Could you check a few things on this model? Use its own coordinates, in mm. A direction names the side the tool comes from. Give positions to 0.01 mm unless a question says otherwise; leave off trailing zeros. Write each loop counter-clockwise with the first axis right and the second up, starting at its lowest first coordinate (ties: lowest second). Pieces come first, ordered by that corner, then holes. Notation, with made-up numbers: (73, 0.25) - (104, 0.25) arc R19 cw to (104, 30.25) - close; hole circle Ø4 at (41.5, -33.75). An arc over 180 degrees is marked (long way). Answer in a Markdown table with one row per item.
Autodesk Inventor part; units mm, degrees
ref_plane "YZ Plane" through (0, 0, 0) normal (1, 0, 0) x (0, 1, 0)
ref_plane "XZ Plane" through (0, 0, 0) normal (0, 1, 0) x (-1, 0, 0)
ref_plane "XY Plane" through (0, 0, 0) normal (0, 0, 1) x (1, 0, 0)
sketch "Sketch1" plane through (0, 0, 0) normal (0, 0, 1) x (1, 0, 0)
  line L0 (33.401, 0) -> (-33.401, 0) construction
  arc A0 (38.9253, 5.6997) -> (35.7349, -7.5866) centre (33.401, 0) ccw construction
  arc A1 (-35.7349, -7.5866) -> (-38.9253, 5.6997) centre (-33.401, 0) ccw construction
  line L1 (19.1135, -12.7) -> (19.1135, -38.1)
  line L2 (-19.1135, -38.1) -> (-19.1135, -12.7)
  line L3 (-19.1135, -12.7) -> (-35.7349, -7.5866)
  arc A2 (35.7349, -7.5866) -> (38.9253, 5.6997) centre (33.401, 0) ccw
  arc A3 (-38.9253, 5.6997) -> (-35.7349, -7.5866) centre (-33.401, 0) ccw
  line L4 (0, 55.245) -> (0, -53.6575) construction
  line L5 (-19.1135, -38.1) -> (19.1135, -38.1)
  line L6 (35.7349, -7.5866) -> (19.1135, -12.7)
  line L7 (38.9253, 5.6997) -> (6.6291, 37.0021)
  circle A4 centre (0, 30.1625) radius 9.525
  line L8 (-6.6291, 37.0021) -> (-38.9253, 5.6997)
  line L9 (29.1304, 6.35) -> (8.6581, 26.1923)
  line L10 (3.175, 21.1822) -> (3.175, 6.35)
  line L11 (3.175, 6.35) -> (29.1304, 6.35)
  line L12 (-29.1304, 6.35) -> (-8.6581, 26.1923)
  line L13 (-3.175, 21.1822) -> (-3.175, 6.35)
  line L14 (-3.175, 6.35) -> (-29.1304, 6.35)
  point P0 (0, 0)
  point P1 (0, 0)
  point P2 (-8.6581, 26.1923)
  point P3 (-3.175, 21.1822)
  dimension "d24" = 50.927
  dimension "d25" = 7.9375
  dimension "d26" = 25.4
  dimension "d30" = 6.35
  dimension "d73" = 12.7
  dimension "d112" = 9.525
  dimension "d113" = 30.1625
  dimension "d115" = 6.35
  dimension "d116" = 6.35
  dimension "d117" = 6.35
extrude "Extrusion2" add sketch "Sketch1" along normal mid plane 9.525 contours L1 L5 L2 L3 A3 L8 A4 L12 L14 L13 L10 L11 L9 L7 A2 L6 | A4
sketch "Sketch2" plane through (0, 0, 4.7625) normal (0, 0, 1) x (1, 0, 0)
  arc A0 (-38.9253, 5.6997) -> (-35.7349, -7.5866) centre (-33.401, 0) ccw construction
  line L0 (-33.401, 0) -> (33.401, 0) construction
  point P0 (0, 0)
  point P1 (0, 0)
hole "Hole1" at (33.401, 0, 4.7625) at (-33.401, 0, 4.7625) direction (0, 0, -1) diameter 3.9624 end through all
sketch "Sketch3" plane through (0, 0, -4.7625) normal (0, 0, -1) x (-1, 0, 0)
  line L0 (-57.8739, 0) -> (57.8739, 0) construction
  line L1 (0, -53.6575) -> (0, 55.245) construction
  line L2 (12.7, -1.5875) -> (-12.7, -1.5875) construction
  line L3 (12.7, -14.2875) -> (-12.7, -14.2875) construction
  line L4 (12.7, -26.9875) -> (-12.7, -26.9875) construction
  point P0 (0, 0)
  point P1 (0, -1.5875)
  point P2 (0, -14.2875)
  point P3 (0, -26.9875)
  dimension "d43" = 25.4
  dimension "d45" = 1.5875
  dimension "d107" = 12.7
hole "Hole2" at (12.7, -1.5875, -4.7625) at (-12.7, -1.5875, -4.7625) at (0, -1.5875, -4.7625) at (12.7, -14.2875, -4.7625) at (0, -14.2875, -4.7625) at (-12.7, -14.2875, -4.7625) at (12.7, -26.9875, -4.7625) at (0, -26.9875, -4.7625) at (-12.7, -26.9875, -4.7625) direction (0, 0, 1) diameter 3.9624 end through all
sketch "Sketch6" plane through (19.1135, -38.1, 4.7625) normal (1, 0, 0) x (0, 0, -1)
  line L0 (9.525, 25.4) -> (0, 25.4) construction
  line L1 (0, 0) -> (0, 25.4) construction
  line L2 (9.525, 25.4) -> (9.525, 0) construction
  line L3 (9.525, 0) -> (0, 0)
  point P0 (4.7625, 38.1)
  point P1 (4.7625, 15.875)
  dimension "d74" = 22.225
hole "Hole3" at (19.1135, -22.225, 0) direction (-1, 0, 0) diameter 3.9624 end through all
sketch "Sketch7" plane through (0, 0, 4.7625) normal (0, 0, 1) x (1, 0, 0)
  arc A0 (6.6291, 37.0021) -> (-6.6291, 37.0021) centre (0, 30.1625) ccw construction
  point P0 (0, 0)
hole "Hole4" at (0, 30.1625, 4.7625) direction (0, 0, -1) diameter 4.9784 end through all
fillet "Fillet5" radius 3.175 2 edges at (-19.1135, -38.1, 0) (19.1135, -38.1, 0)
fillet "Fillet7" radius 1.5875 10 edges at (-19.1135, -12.7, 0) (19.1135, -12.7, 0) (29.1304, 6.35, 0) (3.175, 6.35, 0) (3.175, 21.1822, 0) (8.6581, 26.1923, 0) (-3.175, 21.1822, 0) (-8.6581, 26.1923, 0) (-3.175, 6.35, 0) (-29.1304, 6.35, 0)
equation "\"BendRadius\" = Thickness"
equation "\"BendReliefWidth\" = Thickness"
equation "\"BendReliefDepth\" = 0.5 * Thickness"
equation "\"CornerReliefSize\" = 4 * Thickness"
equation "\"MinimumRemnant\" = 2 * Thickness"
equation "\"TransitionRadius\" = BendRadius"
equation "\"JacobiRadiusSize\" = BendRadius"
equation "\"GapSize\" = Thickness"
properties part number "PLATE,TOP,ELEVATOR,STAGE1" material "Aluminum 7075"
1) If I drill on line 1 (X direction, y = -27, z = -2); line 2 (X direction, y = 13, z = -2) (3 decimals); line 3 (Y direction, x = 13, z = -3.5), over which ranges is the centre line in solid material (lowest first)?
Check values:
| item | result |
|---|---|
| line 1 | x = -19.11 to -14.68, -10.72 to -1.98, 1.98 to 10.72, 14.68 to 19.11 |
| line 2 | x = -31.393 to -22.269, -3.175 to 3.175, 22.269 to 31.393 |
| line 3 | y = -38.1 to -28.95, -25.03 to -16.25, -12.33 to -3.55, 0.37 to 6.35, 21.98 to 30.83 |
2) We'd pull the mould along X, two halves only. Please class faces 3 (the face through (28.09, -9.94, -0.07)), 4 (the face through (6.115, 22.86, -0.067)), 5 (the face through (-3.175, 14, 0)), 6 (the face through (0, -38.1, 0)): +X half, -X half, draft (parallel to the pull), parting line (faces both ways), or undercut.
Check values:
| item | result |
|---|---|
| face 3 | +X half |
| face 4 | undercut |
| face 5 | undercut |
| face 6 | draft |
3) Imagine slicing it at B-B (z = 1). State how many separate pieces and enclosed holes the cut face has, then the cut area to 3 significant figures.
Check values:
| item | result |
|---|---|
| separate pieces | 2 |
| enclosed holes | 14 |
| area | 2,900 mm2 |
4) On a 3-axis mill with a long thin cutter (end or side, diameter ignored), from which of +Z, -Z, +X, -X, +Y, -Y can I reach the whole of each face in a straight line? I mean faces 1 (the face through (15, 6.35, 0)), 2 (the face through (23.003, 21.132, -0.067)). Say none if no direction works.
Check values:
| item | result |
|---|---|
| face 1 | +Z, -Z |
| face 2 | +Z, -Z, +X, +Y |
5) Imagine slicing it at D-D (y = -31). List the corners of the cut face in (x, z) for me, then the cut area to 3 significant figures.
Check values:
| item | result |
|---|---|
| outline | (-19.11, -4.76) - (19.11, -4.76) - (19.11, 4.76) - (-19.11, 4.76) - close |
| area | 364 mm2 |
6) Imagine slicing it at A-A (x = -1). List the corners of the cut face in (y, z) for me (1 decimal).
Check values:
| item | result |
|---|---|
| outline | (-38.1, -4.8) - (-28.7, -4.8) - (-28.7, 4.8) - (-38.1, 4.8) - close; (-25.3, -4.8) - (-16, -4.8) - (-16, 4.8) - (-25.3, 4.8) - close; (-12.6, -4.8) - (-3.3, -4.8) - (-3.3, 4.8) - (-12.6, 4.8) - close; (0.1, -4.8) - (27.9, -4.8) - (27.9, 4.8) - (0.1, 4.8) - close; (32.4, -4.8) - (39.6, -4.8) - (39.6, 4.8) - (32.4, 4.8) - close; hole circle Ø4 at (-22.2, 0) |
7) Will these pins go through, and if not, where does the flat tip stop? P1, Ø3, axis at x = 12.7, y = -14.29, coming from the -Z side; P2, Ø5, axis at y = -22.5, z = -0.5, coming from the +X side.
Check values:
| item | result |
|---|---|
| P1 | passes through |
| P2 | stops at x = 19.11 |
